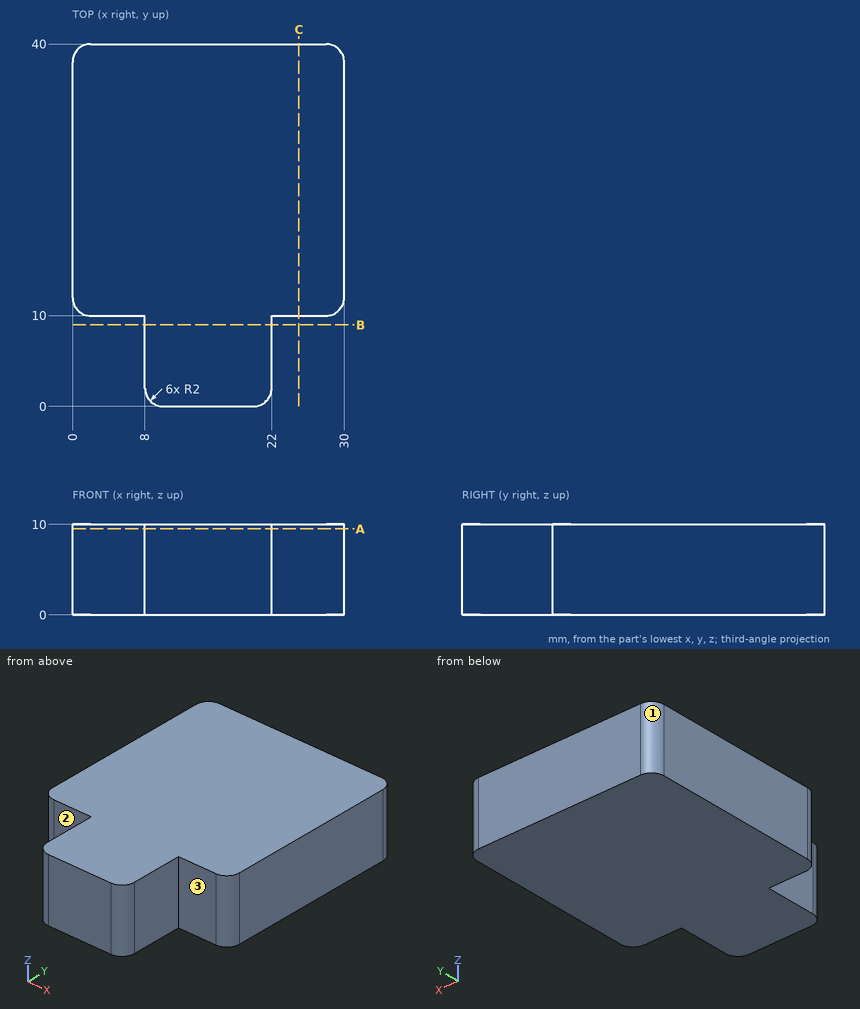
Here's the drawing with two shaded views (mm, measured from the low corner). I have some questions. A direction names the side the tool comes from. Coordinates: 2 decimals unless noted, no trailing zeros. Write each loop counter-clockwise with the first axis right and the second up, starting at its lowest first coordinate (ties: lowest second). Pieces come first, ordered by that corner, then holes. Notation, with made-up numbers: (-38.75, -16.75) -> (-12.75, -16.75) arc R18 ccw to (-12.75, -6.75) -> close; hole circle Ø2 at (36, 85.5). An arc over 180 degrees is marked (long way). One line per question, with ' | ' between items. Start each with the question number.
1. Will these pins go through, and if not, where does the flat tip stop? P1, Ø12, axis at x = 22.5, y = 25.5, coming from the -Z side; P2, Ø3, axis at x = 5, z = 6.5, coming from the -Y side; P3, Ø2.5, axis at y = 5.5, z = 4.5, coming from the -X side; P4, Ø4, axis at y = 6.5, z = 7, coming from the +X side.
2. If we section it at A-A (z = 9.5): Please give me the cut outline in (x, y).
3. If we section it at B-B (y = 9): Please give me the cut outline in (x, z), and give its area (3 significant figures).
4. If we section it at C-C (x = 25): Please give me the cut outline in (y, z), and give its area (3 significant figures).
5. For the marked faces 1, 2 and 3, which set-ups out of +Z, -Z, +X, -X, +Y, -Y let a thin tool reach every point of the face, with its end or its side?
6. Please list where these lines run through material, in increasing order: line 1 along Y through (x, z) = (5.25, 2); line 2 along X through (y, z) = (9, 2.25); line 3 along Y through (x, z) = (28.75, 1.5).
Return value:
1) P1: stops at z = 0 | P2: stops at y = 10 | P3: stops at x = 8 | P4: stops at x = 22
2) outline: (0, 12) arc R2 ccw to (2, 10) -> (8, 10) -> (8, 2) arc R2 ccw to (10, 0) -> (20, 0) arc R2 ccw to (22, 2) -> (22, 10) -> (28, 10) arc R2 ccw to (30, 12) -> (30, 38) arc R2 ccw to (28, 40) -> (2, 40) arc R2 ccw to (0, 38) -> close
3) outline: (8, 0) -> (22, 0) -> (22, 10) -> (8, 10) -> close | area: 140 mm²
4) outline: (10, 0) -> (40, 0) -> (40, 10) -> (10, 10) -> close | area: 300 mm²
5) face 1: +Z, -Z, -X, +Y | face 2: +Z, -Z, -X, -Y | face 3: +Z, -Z, +X, -Y
6) line 1: y = 10 to 40 | line 2: x = 8 to 22 | line 3: y = 10.15 to 39.85
